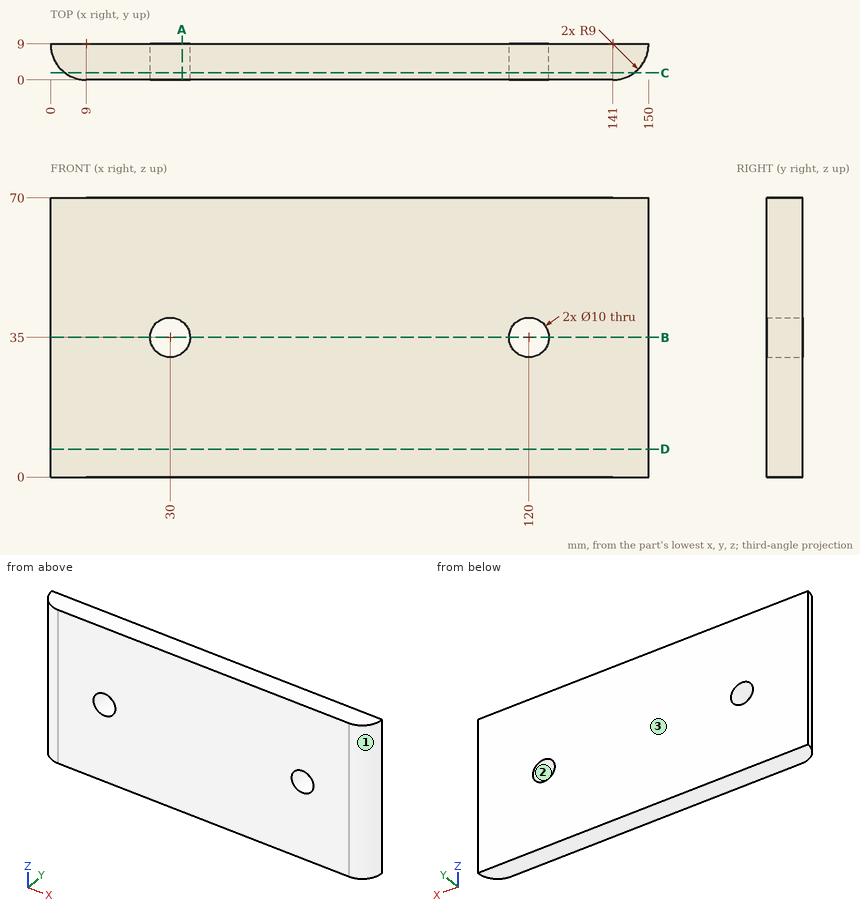
Answer from the drawing. Dimensions are ordinates in mm from the lowest x, y and z of the part. Give positions to 0.01 mm unless a question says otherwise; leave off trailing zeros. Write each loop counter-clockwise with the first axis right and the second up, starting at its lowest first coordinate (ties: lowest second). Pieces come first, ordered by that corner, then holes. Notation, with made-up numbers: (67.5, 58.5) - (81.5, 58.5) arc R26 ccw to (81.5, 76.5) - close; hole circle Ø10 at (-32.75, -9). An arc over 180 degrees is marked (long way). Answer in a Markdown table with one row per item. Add a question column.
Item 1: Find the intervals of material crossed by L1, parallel to Z at x = 120, y = 3.25; L2, parallel to X at y = 2, z = 35; L3, parallel to X at y = 3.5, z = 35, in increasing order.
Item 2: Section D-D, the plane z = 7 is taken. Write down the section's boundary in (x, y).
Item 3: Determine the mould class of the marked faces 1, 2 and 3 for opening direction X: pulls with the +X half, pulls with the -X half, needs draft (parallel to the pull), parting line crosses it, or undercut.
Item 4: Section A-A, the plane x = 33 is taken. Write down the section's boundary in (y, z), and give its area (3 significant figures).
Item 5: Flat-ended cylindrical pins translate along their axes: P1, Ø6, axis at x = 120, z = 35, coming from the -Y side; P2, Ø5, axis at x = 62.5, z = 55, coming from the -Y side; P3, Ø1, axis at y = 1, z = 43.5, coming from the -X side. Find the tip coordinate at first contact, or state that the pin passes through.
Item 6: Section B-B, the plane z = 35 is taken. Write down the section's boundary in (x, y), and give its area (3 significant figures).
Item 7: Section C-C, the plane y = 1.75 is taken. Write down the section's boundary in (x, z).
Recorded:
| question | item | result |
|---|---|---|
| 1 | L1 | z = 0 to 30, 40 to 70 |
| 1 | L2 | x = 3.34 to 25, 35 to 115, 125 to 146.66 |
| 1 | L3 | x = 1.88 to 25, 35 to 115, 125 to 148.12 |
| 2 | outline | (0, 9) arc R9 ccw to (9, 0) - (141, 0) arc R9 ccw to (150, 9) - close |
| 3 | face 1 | pulls with the +X half |
| 3 | face 2 | undercut |
| 3 | face 3 | needs draft |
| 4 | outline | (0, 0) - (9, 0) - (9, 31) - (0, 31) - close; (0, 39) - (9, 39) - (9, 70) - (0, 70) - close |
| 4 | area | 558 mm2 |
| 5 | P1 | passes through |
| 5 | P2 | stops at y = 0 |
| 5 | P3 | stops at x = 4.03 |
| 6 | outline | (0, 9) arc R9 ccw to (9, 0) - (25, 0) - (25, 9) - close; (35, 0) - (115, 0) - (115, 9) - (35, 9) - close; (125, 0) - (141, 0) arc R9 ccw to (150, 9) - (125, 9) - close |
| 6 | area | 1,140 mm2 |
| 7 | outline | (3.67, 0) - (146.33, 0) - (146.33, 70) - (3.67, 70) - close; hole circle Ø10 at (30, 35); hole circle Ø10 at (120, 35) |
